The listing builds one solid part. Answer for the finished solid, in the listing's coordinates (mm). A direction names the side the tool comes from. Coordinates: 2 decimals unless noted, no trailing zeros. Order: outer loops, then holes, each group sorted by start corner. A loop starts at its lowest first (then second) coordinate and runs counter-clockwise, first axis right, second up. Notation, with made-up numbers: (-10.75, 10.5) -> (32.25, 10.5) arc R26 cw to (32.25, 27.5) -> close; hole circle Ø3 at (52.25, 69). An arc over 180 degrees is marked (long way). Write item = value, one per line. Start each with the question number.
```python
from build123d import *

# Parameters (mm, degrees)
BOSS_EXTRUDE1_DEPTH             = 914.4
CUT_EXTRUDE2_REACH              = 14.7
SKETCH3_R                       = 9.525
SKETCH3_R_2                     = 10.31875
F_3_4_0_75_DIAMETER_HOLE1_D     = 19.05
F_3_4_0_75_DIAMETER_HOLE1_DEPTH = 12.7
SKETCH6_R                       = 11.1125
CUT_EXTRUDE3_DEPTH              = 13.7


with BuildPart() as part:
    # Sketch1 → Boss-Extrude1 (new body, symmetric)
    with BuildSketch(Plane.XY):
        with BuildLine():
            Line((0, 0), (0, 152.4))
            Line((0, 152.4), (0.00508, 152.4))
            ThreePointArc((0.00508, 152.4), (8.981744019, 148.681744019), (12.7, 139.70508))
            Line((12.7, 139.70508), (12.7, 25.4))
            ThreePointArc((12.7, 25.4), (16.419743879, 16.419743879), (25.4, 12.7))
            Line((25.4, 12.7), (88.90508, 12.7))
            ThreePointArc((88.90508, 12.7), (97.881744019, 8.981744019), (101.6, 0.00508))
            Line((101.6, 0.00508), (101.6, 0))
            Line((101.6, 0), (0, 0))
        make_face()
    extrude(amount=BOSS_EXTRUDE1_DEPTH, both=True)

    # Sketch3 → Cut-Extrude2 (cut, up to next)
    with BuildSketch(Plane(origin=(0, 12.7, 0), x_dir=(1, 0, 0), z_dir=(0, 1, 0)), mode=Mode.PRIVATE) as cut_extrude2_sk1:
        with Locations((63.5, -863.6)):
            Circle(SKETCH3_R)
    cut_extrude2_tool1 = extrude(cut_extrude2_sk1.sketch, amount=-CUT_EXTRUDE2_REACH, mode=Mode.PRIVATE) & part.part
    add(cut_extrude2_tool1.solids().sort_by_distance((63.5, 12.7, 863.6))[0], mode=Mode.SUBTRACT)
    # Sketch3 → Cut-Extrude2 (cut, up to next)
    with BuildSketch(Plane(origin=(0, 12.7, 0), x_dir=(1, 0, 0), z_dir=(0, 1, 0)), mode=Mode.PRIVATE) as cut_extrude2_sk2:
        with Locations((63.5, 863.6)):
            Circle(SKETCH3_R)
    cut_extrude2_tool2 = extrude(cut_extrude2_sk2.sketch, amount=-CUT_EXTRUDE2_REACH, mode=Mode.PRIVATE) & part.part
    add(cut_extrude2_tool2.solids().sort_by_distance((63.5, 12.7, -863.6))[0], mode=Mode.SUBTRACT)
    # Sketch3 → Cut-Extrude2 (cut, up to next)
    with BuildSketch(Plane(origin=(0, 12.7, 0), x_dir=(1, 0, 0), z_dir=(0, 1, 0)), mode=Mode.PRIVATE) as cut_extrude2_sk3:
        with Locations((63.5, 25.654)):
            Circle(SKETCH3_R_2)
    cut_extrude2_tool3 = extrude(cut_extrude2_sk3.sketch, amount=-CUT_EXTRUDE2_REACH, mode=Mode.PRIVATE) & part.part
    add(cut_extrude2_tool3.solids().sort_by_distance((63.5, 12.7, -25.654))[0], mode=Mode.SUBTRACT)
    # Sketch3 → Cut-Extrude2 (cut, up to next)
    with BuildSketch(Plane(origin=(0, 12.7, 0), x_dir=(1, 0, 0), z_dir=(0, 1, 0)), mode=Mode.PRIVATE) as cut_extrude2_sk4:
        with Locations((63.5, -812.8)):
            Circle(SKETCH3_R)
    cut_extrude2_tool4 = extrude(cut_extrude2_sk4.sketch, amount=-CUT_EXTRUDE2_REACH, mode=Mode.PRIVATE) & part.part
    add(cut_extrude2_tool4.solids().sort_by_distance((63.5, 12.7, 812.8))[0], mode=Mode.SUBTRACT)
    # Sketch3 → Cut-Extrude2 (cut, up to next)
    with BuildSketch(Plane(origin=(0, 12.7, 0), x_dir=(1, 0, 0), z_dir=(0, 1, 0)), mode=Mode.PRIVATE) as cut_extrude2_sk5:
        with Locations((63.5, 711.2)):
            Circle(SKETCH3_R_2)
    cut_extrude2_tool5 = extrude(cut_extrude2_sk5.sketch, amount=-CUT_EXTRUDE2_REACH, mode=Mode.PRIVATE) & part.part
    add(cut_extrude2_tool5.solids().sort_by_distance((63.5, 12.7, -711.2))[0], mode=Mode.SUBTRACT)
    # Sketch3 → Cut-Extrude2 (cut, up to next)
    with BuildSketch(Plane(origin=(0, 12.7, 0), x_dir=(1, 0, 0), z_dir=(0, 1, 0)), mode=Mode.PRIVATE) as cut_extrude2_sk6:
        with Locations((63.5, 457.2)):
            Circle(SKETCH3_R_2)
    cut_extrude2_tool6 = extrude(cut_extrude2_sk6.sketch, amount=-CUT_EXTRUDE2_REACH, mode=Mode.PRIVATE) & part.part
    add(cut_extrude2_tool6.solids().sort_by_distance((63.5, 12.7, -457.2))[0], mode=Mode.SUBTRACT)
    # Sketch3 → Cut-Extrude2 (cut, up to next)
    with BuildSketch(Plane(origin=(0, 12.7, 0), x_dir=(1, 0, 0), z_dir=(0, 1, 0)), mode=Mode.PRIVATE) as cut_extrude2_sk7:
        with Locations((63.5, -228.346)):
            Circle(SKETCH3_R_2)
    cut_extrude2_tool7 = extrude(cut_extrude2_sk7.sketch, amount=-CUT_EXTRUDE2_REACH, mode=Mode.PRIVATE) & part.part
    add(cut_extrude2_tool7.solids().sort_by_distance((63.5, 12.7, 228.346))[0], mode=Mode.SUBTRACT)
    # Sketch3 → Cut-Extrude2 (cut, up to next)
    with BuildSketch(Plane(origin=(0, 12.7, 0), x_dir=(1, 0, 0), z_dir=(0, 1, 0)), mode=Mode.PRIVATE) as cut_extrude2_sk8:
        with Locations((63.5, 362.204)):
            Circle(SKETCH3_R_2)
    cut_extrude2_tool8 = extrude(cut_extrude2_sk8.sketch, amount=-CUT_EXTRUDE2_REACH, mode=Mode.PRIVATE) & part.part
    add(cut_extrude2_tool8.solids().sort_by_distance((63.5, 12.7, -362.204))[0], mode=Mode.SUBTRACT)
    # Sketch3 → Cut-Extrude2 (cut, up to next)
    with BuildSketch(Plane(origin=(0, 12.7, 0), x_dir=(1, 0, 0), z_dir=(0, 1, 0)), mode=Mode.PRIVATE) as cut_extrude2_sk9:
        with Locations((63.5, 108.204)):
            Circle(SKETCH3_R_2)
    cut_extrude2_tool9 = extrude(cut_extrude2_sk9.sketch, amount=-CUT_EXTRUDE2_REACH, mode=Mode.PRIVATE) & part.part
    add(cut_extrude2_tool9.solids().sort_by_distance((63.5, 12.7, -108.204))[0], mode=Mode.SUBTRACT)
    # Sketch3 → Cut-Extrude2 (cut, up to next)
    with BuildSketch(Plane(origin=(0, 12.7, 0), x_dir=(1, 0, 0), z_dir=(0, 1, 0)), mode=Mode.PRIVATE) as cut_extrude2_sk10:
        with Locations((63.5, 812.8)):
            Circle(SKETCH3_R)
    cut_extrude2_tool10 = extrude(cut_extrude2_sk10.sketch, amount=-CUT_EXTRUDE2_REACH, mode=Mode.PRIVATE) & part.part
    add(cut_extrude2_tool10.solids().sort_by_distance((63.5, 12.7, -812.8))[0], mode=Mode.SUBTRACT)

    # 3/4 (0.75) Diameter Hole1
    with Locations(Plane(origin=(12.7, 0, 0), x_dir=(0, 0, -1), z_dir=(1, 0, 0))):
        with Locations((-762, 127)):
            Hole(F_3_4_0_75_DIAMETER_HOLE1_D / 2, depth=F_3_4_0_75_DIAMETER_HOLE1_DEPTH)

    # Sketch6 → Cut-Extrude3 (cut, through all)
    with BuildSketch(Plane(origin=(12.7, 0, 0), x_dir=(0, 0, -1), z_dir=(1, 0, 0))):
        with Locations((-158.496, 127)):
            Circle(SKETCH6_R)
    extrude(amount=-CUT_EXTRUDE3_DEPTH, mode=Mode.SUBTRACT)


solid = part.part
```
Item 1: Which of the six approach directions +Z, -Z, +X, -X, +Y, -Y give full straight-line access (tool end or side, diameter ignored) to faces 1 (the flat face through (57, 12.7, 13)), 2 (the flat face through (0, 75, 13))?
Item 2: Each of these flat-tipped pins is pushed along its axis until it touches: pin 1 (4 mm diameter, centred on y = 16, z = -731, fed in from +X); pin 2 (10 mm diameter, centred on x = 14.5, z = 625, fed in from +Y); pin 3 (6 mm diameter, centred on y = 75, z = 688, fed in from +X). Where does it stop, or does it pass through?
Item 3: Consider probe 1 along X at (y, z) = (42, 692); probe 2 along X at (y, z) = (3, 812.8) (3 decimals). Determine where each line is inside the solid, lowest interval first.
Item 4: Section B-B, the plane y = 47 is taken. Give the vertices of the cut face in (x, z), then the cut area to 3 significant figures.
A:
q1.face_1 = +Z, -Z, +X, +Y
q1.face_2 = +Z, -Z, -X, +Y, -Y
q2.pin_1 = 19.8
q2.pin_2 = 148.13
q2.pin_3 = 12.7
q3.probe_1 = 0 to 12.7
q3.probe_2 = 0 to 53.975, 73.025 to 101.242
q4.outline = (0, -914.4) -> (12.7, -914.4) -> (12.7, 914.4) -> (0, 914.4) -> close
q4.area = 23,200 mm^2
